Could you check a few things on this model? Use its own coordinates, in mm. A direction names the side the tool comes from. Round coordinates to 2 decimals unless told otherwise and drop trailing zeros. Loops run counter-clockwise (first coordinate to the right, second up) from the corner with the lowest first, then second, coordinate; pieces in that order, holes last. Notation, with made-up numbers: (29, -24.5) - (59, -24.5) arc R33 cw to (59, 4.5) - close; hole circle Ø2 at (21.5, 78.5). An arc over 180 degrees is marked (long way). Answer as CSV lines item,"result". Start each with the question number.
1) Suppose I cut it at D-D, the plane z = 0. Write out the boundary of the cut face in (x, y).
2) Which directions (+Z, -Z, +X, -X, +Y, -Y) give clear straight access to the entire face, cutting with the end or side of a thin tool? Please do faces 1 (the face through (47, 0, 9.965)), 2 (the face through (75, -1, 0)), 3 (the face through (47, -5, -15)), 4 (the face through (47, -15, 5)).
3) I'm going to push flat-ended pins straight in: pin 1 Ø4 at (x, y) = (31, 5.5) entering from -Z; pin 2 Ø4.5 at (x, y) = (47, 16) entering from -Z; pin 3 Ø10.5 at (x, y) = (32.5, -13.5) entering from -Z. Where does each tip first touch, or does it pass through?
4) Please list where these lines run through material, in increasing order: line 1 along Z through (x, y) = (85.75, 0); line 2 along Y through (x, z) = (86, 0); line 3 along Z through (x, y) = (59, -14.5).
5) We'd pull the mould along Z, two halves only. Please class faces 5 (the face through (46.835, 14.036, -14.247)), 6 (the face through (47, 15, 5)), 7 (the face through (47, 9.965, 0)), 8 (the face through (47, 5, 15)): pulls with the +Z half, pulls with the -Z half, needs draft (parallel to the pull), parting line crosses it, or undercut.
6) Suppose I cut it at A-A, the plane x = 78. Write out the boundary of the cut face in (y, z) (3 decimals), then the cut area to 3 significant figures.
7) Suppose I cut it at B-B, the plane y = 17. Write out the boundary of the cut face in (x, z), then the cut area to 3 significant figures.
```python
from build123d import *

# Parameters (mm, degrees)
EXTRUDED_CONNECTOR_DEPTH = 95
KEY_CUT_DEPTH            = 20


with BuildPart() as part:
    # Sketch1 → Extruded Connector (new body)
    with BuildSketch(Plane(origin=(0, 0, 0), x_dir=(0, 0, -1), z_dir=(1, 0, 0))):
        with BuildLine():
            ThreePointArc((-19.364916731, -5), (-14.142135624, -14.142135624), (-5, -19.364916731))
            Line((-5, -19.364916731), (-5, -9.964916731))
            Line((-5, -9.964916731), (5, -9.964916731))
            Line((5, -9.964916731), (5, -19.364916731))
            ThreePointArc((5, -19.364916731), (14.142135624, -14.142135624), (19.364916731, -5))
            Line((19.364916731, -5), (9.964916731, -5))
            Line((9.964916731, -5), (9.964916731, 5))
            Line((9.964916731, 5), (19.364916731, 5))
            ThreePointArc((19.364916731, 5), (14.142135624, 14.142135624), (5, 19.364916731))
            Line((5, 19.364916731), (5, 9.964916731))
            Line((5, 9.964916731), (-5, 9.964916731))
            Line((-5, 9.964916731), (-5, 19.364916731))
            ThreePointArc((-5, 19.364916731), (-14.142135624, 14.142135624), (-19.364916731, 5))
            Line((-19.364916731, 5), (-9.964916731, 5))
            Line((-9.964916731, 5), (-9.964916731, -5))
            Line((-9.964916731, -5), (-19.364916731, -5))
        make_face()
    extrude(amount=EXTRUDED_CONNECTOR_DEPTH)

    # Sketch2 → Key Cut (cut)
    with BuildSketch(Plane(origin=(95, 0, 0), x_dir=(0, 0, -1), z_dir=(1, 0, 0))):
        with BuildLine():
            Line((2.754995463, 2.9), (-2.754995463, 2.9))
            ThreePointArc((-2.754995463, 2.9), (-1.577976259, -3.675593955), (4, 0))
            ThreePointArc((4, 0), (3.675593955, 1.577976259), (2.754995463, 2.9))
        make_face()
    extrude(amount=-KEY_CUT_DEPTH, mode=Mode.SUBTRACT)


solid = part.part
```
Filled sheet:
1,outline,"(0, -9.96) - (95, -9.96) - (95, -4) - (75, -4) - (75, 2.9) - (95, 2.9) - (95, 9.96) - (0, 9.96) - close"
2,face 1,"+Z, +X, -X"
2,face 2,"+X"
2,face 3,"-Z, +X, -X"
2,face 4,"+X, -X, -Y"
3,pin 1,"z = -19.36"
3,pin 2,"z = -14.52"
3,pin 3,"z = -18.22"
4,line 1,"-9.96 to -4, 4 to 9.96"
4,line 2,"-9.96 to -4, 2.9 to 9.96"
4,line 3,"-13.77 to -5, 5 to 13.77"
5,face 5,"pulls with the -Z half"
5,face 6,"undercut"
5,face 7,"undercut"
5,face 8,"needs draft"
6,outline,"(-19.365, -5) arc R20 ccw to (-5, -19.365) - (-5, -9.965) - (5, -9.965) - (5, -19.365) arc R20 ccw to (19.365, -5) - (9.965, -5) - (9.965, 5) - (19.365, 5) arc R20 ccw to (5, 19.365) - (5, 9.965) - (-5, 9.965) - (-5, 19.365) arc R20 ccw to (-19.365, 5) - (-9.965, 5) - (-9.965, -5) - close; hole (2.9, -2.755) - (2.9, 2.755) arc R4 ccw (long way) to start"
6,area,"818 mm²"
7,outline,"(0, -10.54) - (95, -10.54) - (95, -5) - (0, -5) - close; (0, 5) - (95, 5) - (95, 10.54) - (0, 10.54) - close"
7,area,"1,050 mm²"
